from build123d import *

# Parameters (mm, degrees)
IZIM1_R                     = 100
IZIM1_R_2                   = 80
IZIM1_R_3                   = 6
Y_KSEKLIK_EKSTR_ZYON1_DEPTH = 7.5
Y_KSEKLIK_EKSTR_ZYON2_DEPTH = 300
Y_KSEKLIK_EKSTR_ZYON3_START = -10
IZIM3_R                     = 100
IZIM3_R_2                   = 80
Y_KSEKLIK_EKSTR_ZYON3_DEPTH = 10
IZIM4_R                     = 5
KES_EKSTR_ZYON1_DEPTH       = 29
IZIM5_R                     = 100
IZIM5_R_2                   = 34
Y_KSEKLIK_EKSTR_ZYON4_DEPTH = 7.5


with BuildPart() as part:
    # izim1 → Y_kseklik-Ekstr_zyon1 (new, symmetric)
    with BuildSketch(Plane(origin=(0, 0, 0), x_dir=(1, 0, 0), z_dir=(0, 1, 0))):
        with Locations(Location((0, 0, 0), (0, 0, 270))):
            Circle(IZIM1_R)
        with Locations(Location((0, 0, 0), (0, 0, 270))):
            Circle(IZIM1_R_2, mode=Mode.SUBTRACT)
        with Locations(Location((62.578950135, 62.578950135, 0), (0, 0, 270))):
            Circle(IZIM1_R_3, mode=Mode.SUBTRACT)
        with Locations(Location((62.578950135, -62.578950135, 0), (0, 0, 270))):
            Circle(IZIM1_R_3, mode=Mode.SUBTRACT)
        with Locations(Location((-62.578950135, -62.578950135, 0), (0, 0, 270))):
            Circle(IZIM1_R_3, mode=Mode.SUBTRACT)
        with Locations(Location((-62.578950135, 62.578950135, 0), (0, 0, 270))):
            Circle(IZIM1_R_3, mode=Mode.SUBTRACT)
    extrude(amount=Y_KSEKLIK_EKSTR_ZYON1_DEPTH, both=True)

    # izim2 → Y_kseklik-Ekstr_zyon2 (add)
    with BuildSketch(Plane.XZ.offset(7.5)):
        with BuildLine():
            Line((-43.571122801, 67.093645436), (-54.463903502, 83.867056795))
            ThreePointArc((-54.463903502, 83.867056795), (0, 100), (54.463903502, 83.867056795))
            Line((54.463903502, 83.867056795), (43.571122801, 67.093645436))
            ThreePointArc((43.571122801, 67.093645436), (0, 80), (-43.571122801, 67.093645436))
        make_face()
        with BuildLine():
            Line((43.571122801, -67.093645436), (54.463903502, -83.867056795))
            ThreePointArc((54.463903502, -83.867056795), (0, -100), (-54.463903502, -83.867056795))
            Line((-54.463903502, -83.867056795), (-43.571122801, -67.093645436))
            ThreePointArc((-43.571122801, -67.093645436), (0, -80), (43.571122801, -67.093645436))
        make_face()
        with BuildLine():
            Line((-67.093645436, 43.571122801), (-83.867056795, 54.463903502))
            ThreePointArc((-83.867056795, 54.463903502), (-100, 0), (-83.867056795, -54.463903502))
            Line((-83.867056795, -54.463903502), (-67.093645436, -43.571122801))
            ThreePointArc((-67.093645436, -43.571122801), (-80, 0), (-67.093645436, 43.571122801))
        make_face()
        with BuildLine():
            Line((67.093645436, -43.571122801), (83.867056795, -54.463903502))
            ThreePointArc((83.867056795, -54.463903502), (100, 0), (83.867056795, 54.463903502))
            Line((83.867056795, 54.463903502), (67.093645436, 43.571122801))
            ThreePointArc((67.093645436, 43.571122801), (80, 0), (67.093645436, -43.571122801))
        make_face()
    extrude(amount=Y_KSEKLIK_EKSTR_ZYON2_DEPTH)

    # izim3 → Y_kseklik-Ekstr_zyon3 (add)
    with BuildSketch(Plane.XZ.offset(307.5).offset(Y_KSEKLIK_EKSTR_ZYON3_START)):
        with Locations(Location((0, 0, 0), (0, 0, 270))):
            Circle(IZIM3_R)
        with Locations(Location((0, 0, 0), (0, 0, 270))):
            Circle(IZIM3_R_2, mode=Mode.SUBTRACT)
    extrude(amount=Y_KSEKLIK_EKSTR_ZYON3_DEPTH)

    # izim4 → Kes-Ekstr_zyon1 (cut)
    with BuildSketch(Plane.XZ.offset(307.5)):
        with Locations(Location((62.932503526, -62.932503526, 0), (0, 0, 270))):
            Circle(IZIM4_R)
        with Locations(Location((-62.932503526, -62.932503526, 0), (0, 0, 270))):
            Circle(IZIM4_R)
        with Locations(Location((-62.932503526, 62.932503526, 0), (0, 0, 270))):
            Circle(IZIM4_R)
        with Locations(Location((62.932503526, 62.932503526, 0), (0, 0, 270))):
            Circle(IZIM4_R)
    extrude(amount=-KES_EKSTR_ZYON1_DEPTH, mode=Mode.SUBTRACT)

    # izim5 → Y_kseklik-Ekstr_zyon4 (add, symmetric)
    with BuildSketch(Plane(origin=(0, -232.5, 0), x_dir=(1, 0, 0), z_dir=(0, 1, 0))):
        with Locations(Location((0, 0, 0), (0, 0, 90))):
            Circle(IZIM5_R)
        with Locations(Location((0, 0, 0), (0, 0, 270))):
            Circle(IZIM5_R_2, mode=Mode.SUBTRACT)
    extrude(amount=Y_KSEKLIK_EKSTR_ZYON4_DEPTH, both=True)


solid = part.part
For this review, take the finished solid that the model builds, in its own axes (mm). A direction names the side the tool comes from. Coordinates: 2 decimals unless noted, no trailing zeros. Order: outer loops, then holes, each group sorted by start corner. A loop starts at its lowest first (then second) coordinate and runs counter-clockwise, first axis right, second up. Notation, with made-up numbers: (87, 7.5) -> (132, 7.5) arc R28 cw to (132, 34.5) -> close; hole circle Ø10 at (-29, 68.25). An arc over 180 degrees is marked (long way). Return JSON: item names as keys, results as strings.
1. We need section B-B on z = 0. Write out the cut boundary in (x, y).
Answer block:
{"outline": "(-100, -307.5) -> (-80, -307.5) -> (-80, -240) -> (-34, -240) -> (-34, -225) -> (-80, -225) -> (-80, 7.5) -> (-100, 7.5) -> close; (34, -240) -> (80, -240) -> (80, -307.5) -> (100, -307.5) -> (100, 7.5) -> (80, 7.5) -> (80, -225) -> (34, -225) -> close"}
2. For pin 1 Ø10 at (x, z) = (-30, 44.5) entering from +Y; pin 2 Ø9 at (x, z) = (-62.93, 62.93) entering from -Y; pin 3 Ø4 at (y, z) = (-207.5, 18.5) entering from +X, all flat-tipped, find the tip position at first contact; note any pin that passes through.
Answer block:
{"pin 1": "y = -225", "pin 2": "y = -240", "pin 3": "x = 98.63"}
3. Machinability: for faces 4 (the cylindrical face through (59.89, -302.57, -58.965)), 5 (the flat face through (49.094, -114.728, 75.598)), 6 (the flat face through (-1, -240, -36)), which of the approach directions +Z, -Z, +X, -X, +Y, -Y give a long, thin tool a straight path to every point of the face, cutting with its end or side? Answer none if there is none.
Answer block:
{"face 4": "-Y", "face 5": "+X", "face 6": "none"}
4. The part is to be moulded in two halves that separate along Z. For faces 1 (the flat face through (75.598, -268.348, 49.094)), 2 (the flat face through (-75.598, -114.728, -49.094)), 3 (the flat face through (-48.94, -268.35, 75.36)), say which applies: +Z half, -Z half, draft (parallel to the pull), parting line (faces both ways), or undercut.
Answer block:
{"face 1": "+Z half", "face 2": "-Z half", "face 3": "undercut"}
5. We need section A-A on y = -129.5. Write out the cut boundary in (x, z).
Answer block:
{"outline": "(-83.87, -54.46) -> (-67.09, -43.57) arc R80 cw to (-67.09, 43.57) -> (-83.87, 54.46) arc R100 ccw to start; (-54.46, -83.87) arc R100 ccw to (54.46, -83.87) -> (43.57, -67.09) arc R80 cw to (-43.57, -67.09) -> close; (-54.46, 83.87) -> (-43.57, 67.09) arc R80 cw to (43.57, 67.09) -> (54.46, 83.87) arc R100 ccw to start; (67.09, -43.57) -> (83.87, -54.46) arc R100 ccw to (83.87, 54.46) -> (67.09, 43.57) arc R80 cw to start"}
6. For line 1 (X direction, y = -232, z = 0); line 2 (Y direction, x = 47, z = -46.5); line 3 (X direction, y = -13, z = -19), list the stretches that pass through material, from the lowest coordinate up. Write a range as from..to.
Answer block:
{"line 1": "-100..-34, 34..100", "line 2": "-240..-225", "line 3": "-98.18..-77.71, 77.71..98.18"}
7. We need section D-D on x = -76. Write out the cut boundary in (y, z).
Answer block:
{"outline": "(-307.5, -64.99) -> (-297.5, -64.99) -> (-297.5, -49.35) -> (-240, -49.35) -> (-240, -64.99) -> (-225, -64.99) -> (-225, -49.35) -> (-7.5, -49.35) -> (-7.5, -64.99) -> (7.5, -64.99) -> (7.5, -24.98) -> (-225, -24.98) -> (-225, 24.98) -> (7.5, 24.98) -> (7.5, 64.99) -> (-7.5, 64.99) -> (-7.5, 49.35) -> (-225, 49.35) -> (-225, 64.99) -> (-240, 64.99) -> (-240, 49.35) -> (-297.5, 49.35) -> (-297.5, 64.99) -> (-307.5, 64.99) -> (-307.5, 24.98) -> (-240, 24.98) -> (-240, -24.98) -> (-307.5, -24.98) -> close"}
